Build history of the part. All positions in model axes, mm. Face numbers are marked on the shaded views. A direction names the side the tool comes from. Give positions to 0.01 mm unless a question says otherwise; leave off trailing zeros. Write each loop counter-clockwise with the first axis right and the second up, starting at its lowest first coordinate (ties: lowest second). Pieces come first, ordered by that corner, then holes. Notation, with made-up numbers: (-22, 28.25) -> (-2, 28.25) arc R25 cw to (-2, 50.25) -> close; hole circle Ø4 at (57, 11). An arc over 180 degrees is marked (long way). One line per question, with ' | ' between items. Start each with the question number.
(1) Pull direction Z, two halves, no side cores. Call the marked faces 1, 2 and 3: released by +Z, released by -Z, zero draft, split by the parting line, or undercut.
(2) Tool access for the marked faces 4 and 5: list every direction of +Z, -Z, +X, -X, +Y, -Y with a clear straight run to the whole face (end or side of a thin tool).
(3) Pin check, flat tips, straight feed: P1, Ø6, axis at x = -86.5, z = -6, coming from the +Y side; P2, Ø3, axis at y = 162, z = -87.5, coming from the -X side; P3, Ø5, axis at x = -58.5, z = 52.5, coming from the -Y side. Stop position of each tip, or through.
(4) Drill centre lines: probe 1 along Z at (x, y) = (-3, 6); probe 2 along Y at (x, z) = (-132.25, 98); probe 3 along Z at (x, y) = (3, 4). Where is each one in solid material? Low to high. Write a range as from..to.
(5) Band-saw the part on B-B, the plane z = -26. Give the cut face in (x, y).
(6) Band-saw the part on A-A, the plane y = 69. Give the cut face in (x, z), and give its area (3 significant figures).
(7) Band-saw the part on C-C, the plane x = -16. Give the cut face in (y, z), and give its area (3 significant figures).
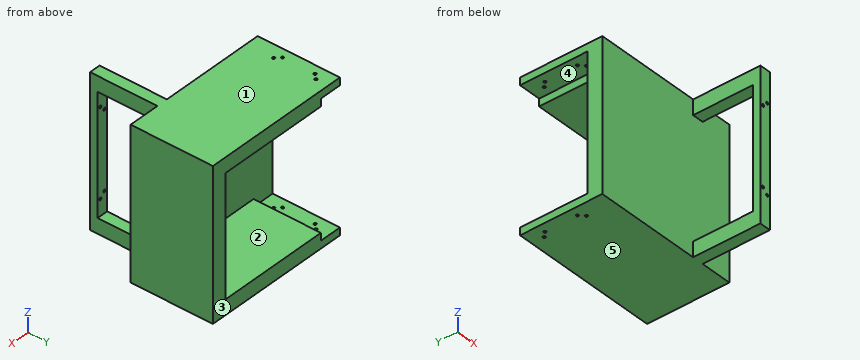
Autodesk Inventor part; units mm, degrees
ref_plane "YZ Plane" through (0, 0, 0) normal (1, 0, 0) x (0, 1, 0)
ref_plane "XZ Plane" through (0, 0, 0) normal (0, 1, 0) x (-1, 0, 0)
ref_plane "XY Plane" through (0, 0, 0) normal (0, 0, 1) x (1, 0, 0)
sketch "Boceto2" plane through (0, 0, 0) normal (0, 1, 0) x (-1, 0, 0)
  line L0 (7.5, 100) -> (-7.5, 100)
  line L1 (-7.5, 100) -> (-7.5, -100)
  line L2 (-7.5, -100) -> (7.5, -100)
  line L3 (7.5, -100) -> (7.5, 100)
  line L4 (7.5, 100) -> (-7.5, -100) construction
  line L5 (-7.5, 100) -> (7.5, -100) construction
  point P0 (0, 0)
  dimension "d7" = 15
  dimension "d8" = 200
extrude "Extrusión1" add sketch "Boceto2" along normal blind 10
sketch "Boceto3" plane through (0, 10, 0) normal (0, 1, 0) x (1, 0, 0)
  circle A0 centre (3.25, 58.25) radius 1.75
  line L0 (5, 50) -> (-5, 50)
  line L1 (-5, 50) -> (-5, 60)
  line L2 (-5, 60) -> (5, 60)
  line L3 (5, 60) -> (5, 50)
  line L4 (5, 50) -> (-5, 60) construction
  line L5 (-5, 50) -> (5, 60) construction
  circle A1 centre (-3.25, 51.75) radius 1.75
  line L6 (7.5, 100) -> (-7.5, 100)
  line L7 (-7.5, 0) -> (3.408, 0)
  line L8 (5, -60) -> (5, -50)
  line L9 (-5, -60) -> (5, -60)
  line L10 (5, -50) -> (-5, -50)
  line L11 (-5, -50) -> (-5, -60)
  line L12 (-5, -50) -> (5, -60) construction
  circle A2 centre (-3.25, -51.75) radius 1.75
  line L13 (5, -50) -> (-5, -60) construction
  circle A3 centre (3.25, -58.25) radius 1.75
  line L14 (-7.5, -100) -> (7.5, -100)
  point P0 (0, 0)
  point P1 (-5, 55)
  point P2 (0, 100)
  point P3 (-5, -55)
  dimension "d11" = 3.5
  dimension "d12" = 1.75
  dimension "d13" = 1.75
  dimension "d14" = 1.75
  dimension "d15" = 1.75
  dimension "d16" = 10
  dimension "d17" = 10
  dimension "d19" = 40
  dimension "d81" = 40
hole "Agujero1" at (3.25, 10, 58.25) at (-3.25, 10, 51.75) at (3.25, 10, -58.25) at (-3.25, 10, -51.75) direction (0, -1, 0) diameter 3.5 end through all
sketch "Boceto4" plane through (0, 10, 0) normal (0, 1, 0) x (1, 0, 0)
  line L0 (-7.5, 100) -> (-7.5, -100)
  line L1 (-7.5, -100) -> (7.5, -100)
  line L2 (7.5, -100) -> (7.5, -80)
  line L3 (7.5, -80) -> (-7.5, -80)
  line L4 (-7.5, -80) -> (-7.5, -100)
  line L5 (-7.5, 0) -> (1.0116, 0)
  line L6 (-7.5, -100) -> (-7.5, 100)
  line L7 (-7.5, 100) -> (7.5, 100)
  line L8 (7.5, 100) -> (7.5, 80)
  line L9 (7.5, 80) -> (-7.5, 80)
  line L10 (-7.5, 80) -> (-7.5, 100)
  point P0 (0, 0)
  point P1 (-7.5, -80)
  point P2 (-7.5, 80)
  dimension "d27" = 15
  dimension "d28" = 20
extrude "Extrusión2" add sketch "Boceto4" along normal blind 80
sketch "Boceto5" plane through (0, 90, 0) normal (0, 1, 0) x (1, 0, 0)
  line L0 (-7.5, -100) -> (7.5, -100)
  line L1 (-7.5, -100) -> (49.5, -100)
  line L2 (49.5, -100) -> (49.5, 100)
  line L3 (49.5, 100) -> (-7.5, 100)
  line L4 (-7.5, 100) -> (-7.5, -100)
  line L5 (49.5, -100) -> (-150.5, -100)
  line L6 (-150.5, -100) -> (-150.5, 100)
  line L7 (-150.5, 100) -> (49.5, 100)
  line L8 (49.5, 100) -> (49.5, -100)
  point P0 (0, 0)
  point P1 (-7.5, 100)
  dimension "d31" = 57
  dimension "d32" = 200
  dimension "d75" = 200
extrude "Extrusión3" add sketch "Boceto5" along normal blind 110
sketch "Boceto6" plane through (0, 200, 0) normal (0, 1, 0) x (1, 0, 0)
  line L0 (49.5, 100) -> (7.5, 100)
  line L1 (49.5, 100) -> (29.5, 100)
  line L2 (29.5, 100) -> (29.5, 80)
  line L3 (7.5, -100) -> (49.5, -100)
  line L4 (28.5, -100) -> (28.5, -80)
  line L5 (-150.5, 100) -> (-150.5, -100)
  line L6 (29.5, 80) -> (-150.5, 80)
  line L7 (-150.5, 80) -> (-150.5, -80)
  line L8 (-150.5, -80) -> (29.5, -80)
  line L9 (29.5, -80) -> (29.5, 80)
  line L10 (-150.5, -100) -> (49.5, -100)
  point P0 (7.5, 80)
  point P1 (-50.5, -100)
  dimension "d36" = 20
  dimension "d37" = 20
  dimension "d38" = 20
  dimension "d77" = 20
extrude "Extrusión4" cut sketch "Boceto6" against normal blind 90 contours L8 L5 L6 L9
sketch "Boceto7" plane through (-150.5, 90, -100) normal (-1, 0, 0) x (0, 0, 1)
  line L0 (0, 110) -> (20, 110)
  line L1 (20, 110) -> (10, 110)
  line L2 (10, 110) -> (10, 20)
  line L3 (10, 20) -> (20, 20)
  line L4 (20, 20) -> (20, 110)
  line L5 (180, 110) -> (180, 20)
  line L6 (180, 110) -> (190, 110)
  line L7 (190, 110) -> (190, 20)
  line L8 (190, 20) -> (180, 20)
  line L9 (180, 20) -> (180, 110)
  line L10 (200, 0) -> (200, 110)
  line L11 (0, 0) -> (0, 110)
  line L12 (0, 110) -> (10, 110)
  line L13 (10, 110) -> (10, 20)
  line L14 (10, 20) -> (0, 20)
  line L15 (0, 20) -> (0, 110)
  line L16 (200, 110) -> (0, 110)
  line L17 (200, 110) -> (190, 110)
  line L18 (190, 110) -> (190, 20)
  line L19 (190, 20) -> (200, 20)
  line L20 (200, 20) -> (200, 110)
  point P0 (100, -90)
  dimension "d63" = 10
  dimension "d65" = 10
  dimension "d76" = 10
extrude "Extrusión5" cut sketch "Boceto7" against normal blind 30 contours L6 L7 L8 L5 | L0 L4 L3 L2
sketch "Boceto8" plane through (-7.5, 0, 100) normal (0, 0, 1) x (1, 0, 0)
  line L0 (-113, 110) -> (-113, 200)
  line L1 (-113, 200) -> (-113, 110)
  circle A0 centre (-124.75, 183.25) radius 1.75
  line L2 (-123, 175) -> (-133, 175)
  line L3 (-133, 175) -> (-133, 185)
  line L4 (-133, 185) -> (-123, 185)
  line L5 (-123, 185) -> (-123, 175)
  line L6 (-123, 175) -> (-133, 185) construction
  line L7 (-133, 175) -> (-123, 185) construction
  circle A1 centre (-131.25, 176.75) radius 1.75
  line L8 (-143, 200) -> (57, 200)
  line L9 (-143, 90) -> (-143, 200)
  line L10 (-113, 155) -> (-128, 155)
  line L11 (-123, 125) -> (-123, 135)
  line L12 (-133, 125) -> (-123, 125)
  line L13 (-123, 135) -> (-133, 125) construction
  line L14 (-123, 135) -> (-133, 135)
  line L15 (-133, 135) -> (-123, 125) construction
  circle A2 centre (-131.25, 133.25) radius 1.75
  line L16 (-133, 135) -> (-133, 125)
  circle A3 centre (-124.75, 126.75) radius 1.75
  line L17 (-143, 110) -> (-113, 110)
  point P0 (7.5, 0)
  point P1 (-133, 180)
  point P2 (-123, 180)
  point P3 (-133, 130)
  point P4 (-123, 130)
  dimension "d45" = 3.5
  dimension "d46" = 1.75
  dimension "d47" = 1.75
  dimension "d48" = 1.75
  dimension "d49" = 1.75
  dimension "d50" = 10
  dimension "d51" = 10
  dimension "d52" = 15
  dimension "d53" = 10
  dimension "d54" = 10
  dimension "d55" = 15
hole "Agujero2" at (-132.25, 183.25, 100) at (-138.75, 176.75, 100) at (-138.75, 133.25, 100) at (-132.25, 126.75, 100) direction (0, 0, -1) diameter 3.5 end through all
properties part number "container_front"
Results:
1) face 1: released by +Z | face 2: undercut | face 3: zero draft
2) face 4: -X, +Y | face 5: -Z, +X, -X, +Y, -Y
3) P1: stops at y = 110 | P2: stops at x = -120.5 | P3: stops at y = 90
4) probe 1: z = -100..-53.48, -50.02..50.02, 53.48..100 | probe 2: y = 90..125, 128.5..181.5, 185..200 | probe 3: z = -100..-59.98, -56.52..56.52, 59.98..100
5) outline: (-150.5, 90) -> (49.5, 90) -> (49.5, 200) -> (29.5, 200) -> (29.5, 110) -> (-150.5, 110) -> close; (-7.5, 0) -> (7.5, 0) -> (7.5, 10) -> (-7.5, 10) -> close
6) outline: (-7.5, -100) -> (7.5, -100) -> (7.5, -80) -> (-7.5, -80) -> close; (-7.5, 80) -> (7.5, 80) -> (7.5, 100) -> (-7.5, 100) -> close | area: 600 mm²
7) outline: (90, -100) -> (200, -100) -> (200, -80) -> (110, -80) -> (110, 80) -> (200, 80) -> (200, 100) -> (90, 100) -> close | area: 7,600 mm²
